```python
from build123d import *

# Parameters (mm, degrees)
F0_R     = 38.7121
F0_R_2   = 6
F0_R_3   = 0.75
F0_R_4   = 12.5
F0_R_5   = 4.5
F1_DEPTH = 7
F2_R     = 39.25
F2_R_2   = 38.7121
F2_R_3   = 6
F2_R_4   = 0.75
F2_R_5   = 12.5
F2_R_6   = 4.5
F3_DEPTH = 1
F4_R     = 39.25
F4_R_2   = 38.7121
F4_R_3   = 6
F4_R_4   = 0.75
F4_R_5   = 12.5
F4_R_6   = 4.5
F5_DEPTH = 1
F6_SIZE  = 0.5


with BuildPart() as f1:
    # F0 (on Top) → F1 (new body)
    with BuildSketch(Plane.XY):
        Circle(F0_R)
        with Locations((-21.2132034356, -21.2132034356)):
            Circle(F0_R_2, mode=Mode.SUBTRACT)
        with Locations((-11.6672618896, -11.6672618896)):
            Circle(F0_R_3, mode=Mode.SUBTRACT)
        with Locations((-9.545941546, -9.545941546)):
            Circle(F0_R_3, mode=Mode.SUBTRACT)
        with Locations((-7.4246212025, -7.4246212025)):
            Circle(F0_R_3, mode=Mode.SUBTRACT)
        with Locations((-5.3033008589, -5.3033008589)):
            Circle(F0_R_3, mode=Mode.SUBTRACT)
        with Locations((0, -22)):
            Circle(F0_R_4, mode=Mode.SUBTRACT)
        with Locations((21.2132034356, -21.2132034356)):
            Circle(F0_R_2, mode=Mode.SUBTRACT)
        with Locations((11.6672618896, -11.6672618896)):
            Circle(F0_R_3, mode=Mode.SUBTRACT)
        with Locations((9.545941546, -9.545941546)):
            Circle(F0_R_3, mode=Mode.SUBTRACT)
        with Locations((7.4246212025, -7.4246212025)):
            Circle(F0_R_3, mode=Mode.SUBTRACT)
        with Locations((5.3033008589, -5.3033008589)):
            Circle(F0_R_3, mode=Mode.SUBTRACT)
        with Locations((-22, 0)):
            Circle(F0_R_4, mode=Mode.SUBTRACT)
        with Locations((-5.3033008589, 5.3033008589)):
            Circle(F0_R_3, mode=Mode.SUBTRACT)
        with Locations((-7.4246212025, 7.4246212025)):
            Circle(F0_R_3, mode=Mode.SUBTRACT)
        with Locations((-9.545941546, 9.545941546)):
            Circle(F0_R_3, mode=Mode.SUBTRACT)
        with Locations((-11.6672618896, 11.6672618896)):
            Circle(F0_R_3, mode=Mode.SUBTRACT)
        with Locations((-21.2132034356, 21.2132034356)):
            Circle(F0_R_2, mode=Mode.SUBTRACT)
        Circle(F0_R_5, mode=Mode.SUBTRACT)
        with Locations((5.3033008589, 5.3033008589)):
            Circle(F0_R_3, mode=Mode.SUBTRACT)
        with Locations((7.4246212025, 7.4246212025)):
            Circle(F0_R_3, mode=Mode.SUBTRACT)
        with Locations((9.545941546, 9.545941546)):
            Circle(F0_R_3, mode=Mode.SUBTRACT)
        with Locations((11.6672618896, 11.6672618896)):
            Circle(F0_R_3, mode=Mode.SUBTRACT)
        with Locations((22, 0)):
            Circle(F0_R_4, mode=Mode.SUBTRACT)
        with Locations((0, 22)):
            Circle(F0_R_4, mode=Mode.SUBTRACT)
        with Locations((21.2132034356, 21.2132034356)):
            Circle(F0_R_2, mode=Mode.SUBTRACT)
    extrude(amount=F1_DEPTH)

    # F2 (on face) → F3 (join)
    with BuildSketch(Plane.XY.offset(7)):
        Circle(F2_R)
        Circle(F2_R_2, mode=Mode.SUBTRACT)
        Circle(F2_R_2)
        with Locations((-21.2132034356, -21.2132034356)):
            Circle(F2_R_3, mode=Mode.SUBTRACT)
        with Locations((-11.6672618896, -11.6672618896)):
            Circle(F2_R_4, mode=Mode.SUBTRACT)
        with Locations((-9.545941546, -9.545941546)):
            Circle(F2_R_4, mode=Mode.SUBTRACT)
        with Locations((-7.4246212025, -7.4246212025)):
            Circle(F2_R_4, mode=Mode.SUBTRACT)
        with Locations((-5.3033008589, -5.3033008589)):
            Circle(F2_R_4, mode=Mode.SUBTRACT)
        with Locations((0, -22)):
            Circle(F2_R_5, mode=Mode.SUBTRACT)
        with Locations((21.2132034356, -21.2132034356)):
            Circle(F2_R_3, mode=Mode.SUBTRACT)
        with Locations((11.6672618896, -11.6672618896)):
            Circle(F2_R_4, mode=Mode.SUBTRACT)
        with Locations((9.545941546, -9.545941546)):
            Circle(F2_R_4, mode=Mode.SUBTRACT)
        with Locations((7.4246212025, -7.4246212025)):
            Circle(F2_R_4, mode=Mode.SUBTRACT)
        with Locations((5.3033008589, -5.3033008589)):
            Circle(F2_R_4, mode=Mode.SUBTRACT)
        with Locations((-22, 0)):
            Circle(F2_R_5, mode=Mode.SUBTRACT)
        with Locations((-5.3033008589, 5.3033008589)):
            Circle(F2_R_4, mode=Mode.SUBTRACT)
        with Locations((-7.4246212025, 7.4246212025)):
            Circle(F2_R_4, mode=Mode.SUBTRACT)
        with Locations((-9.545941546, 9.545941546)):
            Circle(F2_R_4, mode=Mode.SUBTRACT)
        with Locations((-11.6672618896, 11.6672618896)):
            Circle(F2_R_4, mode=Mode.SUBTRACT)
        with Locations((-21.2132034356, 21.2132034356)):
            Circle(F2_R_3, mode=Mode.SUBTRACT)
        Circle(F2_R_6, mode=Mode.SUBTRACT)
        with Locations((5.3033008589, 5.3033008589)):
            Circle(F2_R_4, mode=Mode.SUBTRACT)
        with Locations((7.4246212025, 7.4246212025)):
            Circle(F2_R_4, mode=Mode.SUBTRACT)
        with Locations((9.545941546, 9.545941546)):
            Circle(F2_R_4, mode=Mode.SUBTRACT)
        with Locations((11.6672618896, 11.6672618896)):
            Circle(F2_R_4, mode=Mode.SUBTRACT)
        with Locations((22, 0)):
            Circle(F2_R_5, mode=Mode.SUBTRACT)
        with Locations((0, 22)):
            Circle(F2_R_5, mode=Mode.SUBTRACT)
        with Locations((21.2132034356, 21.2132034356)):
            Circle(F2_R_3, mode=Mode.SUBTRACT)
    extrude(amount=F3_DEPTH)

    # F4 (on face) → F5 (join)
    with BuildSketch(Plane(origin=(0, 0, 0), x_dir=(1, 0, 0), z_dir=(0, 0, -1))):
        Circle(F4_R)
        Circle(F4_R_2, mode=Mode.SUBTRACT)
        Circle(F4_R_2)
        with Locations((-21.2132034356, -21.2132034356)):
            Circle(F4_R_3, mode=Mode.SUBTRACT)
        with Locations((-11.6672618896, -11.6672618896)):
            Circle(F4_R_4, mode=Mode.SUBTRACT)
        with Locations((-9.545941546, -9.545941546)):
            Circle(F4_R_4, mode=Mode.SUBTRACT)
        with Locations((-7.4246212025, -7.4246212025)):
            Circle(F4_R_4, mode=Mode.SUBTRACT)
        with Locations((-5.3033008589, -5.3033008589)):
            Circle(F4_R_4, mode=Mode.SUBTRACT)
        with Locations((0, -22)):
            Circle(F4_R_5, mode=Mode.SUBTRACT)
        with Locations((21.2132034356, -21.2132034356)):
            Circle(F4_R_3, mode=Mode.SUBTRACT)
        with Locations((11.6672618896, -11.6672618896)):
            Circle(F4_R_4, mode=Mode.SUBTRACT)
        with Locations((9.545941546, -9.545941546)):
            Circle(F4_R_4, mode=Mode.SUBTRACT)
        with Locations((7.4246212025, -7.4246212025)):
            Circle(F4_R_4, mode=Mode.SUBTRACT)
        with Locations((5.3033008589, -5.3033008589)):
            Circle(F4_R_4, mode=Mode.SUBTRACT)
        with Locations((-22, 0)):
            Circle(F4_R_5, mode=Mode.SUBTRACT)
        with Locations((-5.3033008589, 5.3033008589)):
            Circle(F4_R_4, mode=Mode.SUBTRACT)
        with Locations((-7.4246212025, 7.4246212025)):
            Circle(F4_R_4, mode=Mode.SUBTRACT)
        with Locations((-9.545941546, 9.545941546)):
            Circle(F4_R_4, mode=Mode.SUBTRACT)
        with Locations((-11.6672618896, 11.6672618896)):
            Circle(F4_R_4, mode=Mode.SUBTRACT)
        with Locations((-21.2132034356, 21.2132034356)):
            Circle(F4_R_3, mode=Mode.SUBTRACT)
        Circle(F4_R_6, mode=Mode.SUBTRACT)
        with Locations((5.3033008589, 5.3033008589)):
            Circle(F4_R_4, mode=Mode.SUBTRACT)
        with Locations((7.4246212025, 7.4246212025)):
            Circle(F4_R_4, mode=Mode.SUBTRACT)
        with Locations((9.545941546, 9.545941546)):
            Circle(F4_R_4, mode=Mode.SUBTRACT)
        with Locations((11.6672618896, 11.6672618896)):
            Circle(F4_R_4, mode=Mode.SUBTRACT)
        with Locations((22, 0)):
            Circle(F4_R_5, mode=Mode.SUBTRACT)
        with Locations((0, 22)):
            Circle(F4_R_5, mode=Mode.SUBTRACT)
        with Locations((21.2132034356, 21.2132034356)):
            Circle(F4_R_3, mode=Mode.SUBTRACT)
    extrude(amount=F5_DEPTH)

    # F6
    f6_edges = [f1.edges().sort_by_distance(p)[0] for p in [
        (-39.25, 0, 0),
        (-39.25, 0, 7),
    ]]
    chamfer(f6_edges, length=F6_SIZE)


solid = f1.part
```
Here's how the part is built. I have some questions about the finished solid (model axes, mm). Coordinates: 2 decimals unless noted, no trailing zeros. Use a Markdown table: item, result. Add a question column.
(1) If we section it at A-A, the plane x = 0: State how many separate pieces and enclosed holes the cut face has, and give its area (3 significant figures).
(2) We'd pull the mould along Z, two halves only. Please class faces 1 (the flat face through (-1, 8, -1)), 2 (the cylindrical face through (-38.675, 1.702, 3.451)), 3 (the cylindrical face through (26.756, 23.511, 3.563)): +Z half, -Z half, draft (parallel to the pull), parting line (faces both ways), or undercut.
(3) I'm going to push flat-ended pins straight in: P1, Ø1, axis at y = 21.5, z = 3, coming from the +X side; P2, Ø2, axis at x = -17.5, z = 1.5, coming from the -Y side; P3, Ø1, axis at y = 2.5, z = 1.5, coming from the +X side. Where does each tip first touch, or does it pass through?
(4) Please list where these lines run through material, in increasing order: line 1 (Y direction, x = 0, z = 2); line 2 (X direction, y = -22, z = 4.5); line 3 (X direction, y = 1, z = 4.25).
Outcome:
| question | item | result |
|---|---|---|
| 1 | separate pieces | 4 |
| 1 | enclosed holes | 0 |
| 1 | area | 167 mm^2 |
| 2 | face 1 | -Z half |
| 2 | face 2 | undercut |
| 2 | face 3 | draft |
| 3 | P1 | stops at x = 32.52 |
| 3 | P2 | stops at y = -35.02 |
| 3 | P3 | stops at x = 38.66 |
| 4 | line 1 | y = -38.71 to -34.5, -9.5 to -4.5, 4.5 to 9.5, 34.5 to 38.71 |
| 4 | line 2 | x = -31.85 to -27.16, -15.27 to -12.5, 12.5 to 15.27, 27.16 to 31.85 |
| 4 | line 3 | x = -38.7 to -34.46, -9.54 to -4.39, 4.39 to 9.54, 34.46 to 38.7 |
